```python
from build123d import *

# Parameters (mm, degrees)
EXTRUDE_1_DEPTH     = 11
CUT_EXTRUDE_2_DEPTH = 5


with BuildPart() as part:
    # 草图2 → 凸台-拉伸1 (new body)
    with BuildSketch(Plane(origin=(0, 0, 0), x_dir=(1, 0, 0), z_dir=(0, 1, 0))):
        with BuildLine():
            Line((-12, 9), (0, 9))
            Line((0, 9), (12, 9))
            ThreePointArc((12, 9), (0, 15), (-12, 9))
        make_face()
    extrude(amount=EXTRUDE_1_DEPTH)

    # 草图3 → 切除-拉伸2 (cut)
    with BuildSketch(Plane.XY.offset(-9)):
        with BuildLine():
            ThreePointArc((0, 8), (-2.5, 5.5), (0, 3))
            Line((0, 3), (0, 8))
        make_face()
        with BuildLine():
            Line((0, 8), (0, 3))
            ThreePointArc((0, 3), (1.767766953, 3.732233047), (2.5, 5.5))
            ThreePointArc((2.5, 5.5), (1.767766953, 7.267766953), (0, 8))
        make_face()
    extrude(amount=-CUT_EXTRUDE_2_DEPTH, mode=Mode.SUBTRACT)


solid = part.part
```
Work out the finished part from the listing and answer in its coordinate system (mm). Round coordinates to 2 decimals unless told otherwise and drop trailing zeros. Write each loop counter-clockwise with the first axis right and the second up, starting at its lowest first coordinate (ties: lowest second). Pieces come first, ordered by that corner, then holes.
1) A cutting plane is placed at B-B on y = 3.5. Determine the outline of the cut face in (x, z), and give its area (3 significant figures).
2) A cutting plane is placed at C-C on x = 6. Determine the outline of the cut face in (y, z), and give its area (3 significant figures).
3) A cutting plane is placed at D-D on z = -13.05. Determine the outline of the cut face in (x, y).
4) A cutting plane is placed at A-A on z = -11.7. Determine the outline of the cut face in (x, y), and give its area (3 significant figures).
5) Consider probe 1 along X at (y, z) = (7.25, -12.35); probe 2 along Z at (x, y) = (0.25, 5.5); probe 3 along Y at (x, z) = (0.5, -9.6). Determine where each line is inside the solid, lowest interval first.
6) Determine the mould class of faces 1 (the face through (0, 6, -14)), 2 (the face through (-3, 5, -9)), 3 (the face through (0, 5, -15)) for opening direction X: pulls with the +X half, pulls with the -X half, needs draft (parallel to the pull), parting line crosses it, or undercut.
7) Flat-ended cylindrical pins translate along their axes: P1, Ø1, axis at x = -6.5, z = -12, coming from the -Y side; P2, Ø4, axis at x = 9, y = 6, coming from the -Z side; P3, Ø1.5, axis at x = 0, y = 5, coming from the +Z side; P4, Ø3, axis at y = 7, z = -10, coming from the -X side. Find the tip coordinate at first contact, or state that the pin passes through.
Entries:
1. outline: (-12, -9) arc R15 ccw to (12, -9) - (1.5, -9) - (1.5, -14) - (-1.5, -14) - (-1.5, -9) - close
1. area: 85.6 mm2
2. outline: (0, -13.75) - (11, -13.75) - (11, -9) - (0, -9) - close
2. area: 52.2 mm2
3. outline: (-7.4, 0) - (7.4, 0) - (7.4, 11) - (-7.4, 11) - close; hole circle Ø5 at (0, 5.5)
4. outline: (-9.39, 0) - (9.39, 0) - (9.39, 11) - (-9.39, 11) - close; hole circle Ø5 at (0, 5.5)
4. area: 187 mm2
5. probe 1: x = -8.51 to -1.79, 1.79 to 8.51
5. probe 2: z = -15 to -14
5. probe 3: y = 0 to 3.05, 7.95 to 11
6. face 1: undercut
6. face 2: needs draft
6. face 3: parting line crosses it
7. P1: stops at y = 0
7. P2: stops at z = -13.27
7. P3: stops at z = -14
7. P4: stops at x = -12
